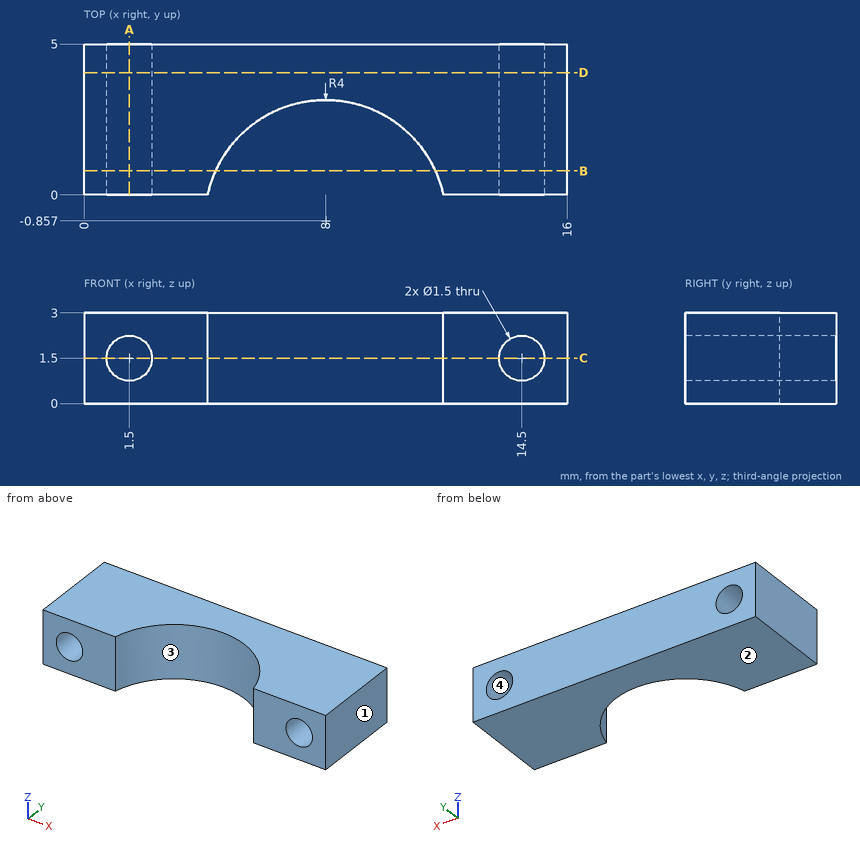
Geometry check sheet. Reference: drawing and pictorial views, mm from the part's lowest x, y, z. Round coordinates to 2 decimals unless told otherwise and drop trailing zeros. Loops run counter-clockwise (first coordinate to the right, second up) from the corner with the lowest first, then second, coordinate; pieces in that order, holes last. Notation, with made-up numbers: (5.5, -28.75) -> (42.5, -28.75) arc R18 cw to (42.5, -6.75) -> close; hole circle Ø10 at (49, 50.25). An arc over 180 degrees is marked (long way). Answer as a JSON object with one key per item and string values.
Q1. Section check B-B (y = 0.8). Record the boundary of the cut face in (x, z).
Data:
{"outline": "(0, 0) -> (4.36, 0) -> (4.36, 3) -> (0, 3) -> close; (11.64, 0) -> (16, 0) -> (16, 3) -> (11.64, 3) -> close; hole circle Ø1.5 at (1.5, 1.5); hole circle Ø1.5 at (14.5, 1.5)"}
Q2. Section check D-D (y = 4.05). Record the boundary of the cut face in (x, z), then the cut area to 3 significant figures.
Data:
{"outline": "(0, 0) -> (16, 0) -> (16, 3) -> (0, 3) -> close; hole circle Ø1.5 at (1.5, 1.5); hole circle Ø1.5 at (14.5, 1.5)", "area": "44.5 mm2"}
Q3. Section check A-A (x = 1.5). Record the boundary of the cut face in (y, z), then the cut area to 3 significant figures.
Data:
{"outline": "(0, 0) -> (5, 0) -> (5, 0.75) -> (0, 0.75) -> close; (0, 2.25) -> (5, 2.25) -> (5, 3) -> (0, 3) -> close", "area": "7.50 mm2"}
Q4. Scan lines: line 1 (Z direction, x = 14.5, y = 3.05); line 2 (X direction, y = 0.8, z = 1.9); line 3 (X direction, y = 1.8, z = 1.65). Record each from-to range of solid material in increasing order. Write a range as from..to.
Data:
{"line 1": "z = 0..0.75, 2.25..3", "line 2": "x = 0..0.87, 2.13..4.36, 11.64..13.87, 15.13..16", "line 3": "x = 0..0.77, 2.23..5.01, 10.99..13.77, 15.23..16"}
Q5. Section check C-C (z = 1.5). Record the boundary of the cut face in (x, y).
Data:
{"outline": "(0, 0) -> (0.75, 0) -> (0.75, 5) -> (0, 5) -> close; (2.25, 0) -> (4.09, 0) arc R4 cw to (11.91, 0) -> (13.75, 0) -> (13.75, 5) -> (2.25, 5) -> close; (15.25, 0) -> (16, 0) -> (16, 5) -> (15.25, 5) -> close"}
Q6. Draft check along X on the marked faces 1, 2, 3 and 4. Enter one of: pulls with the +X half, pulls with the -X half, needs draft (parallel to the pull), parting line crosses it, or undercut.
Data:
{"face 1": "pulls with the +X half", "face 2": "needs draft", "face 3": "undercut", "face 4": "undercut"}
